Can you work these out from the model? Positions are in its coordinate system, mm. Coordinates: 2 decimals unless noted, no trailing zeros. Write each loop counter-clockwise with the first axis right and the second up, starting at its lowest first coordinate (ties: lowest second). Pieces come first, ordered by that corner, then holes. Notation, with made-up numbers: M 29.5,45.25 L 33.5,45.25 A14 ccw 33.5,64.25 Z; hole C 50.5,65.25 d9. An arc over 180 degrees is marked long. Answer as a JSON object with one key per item and string values. Group by question number.
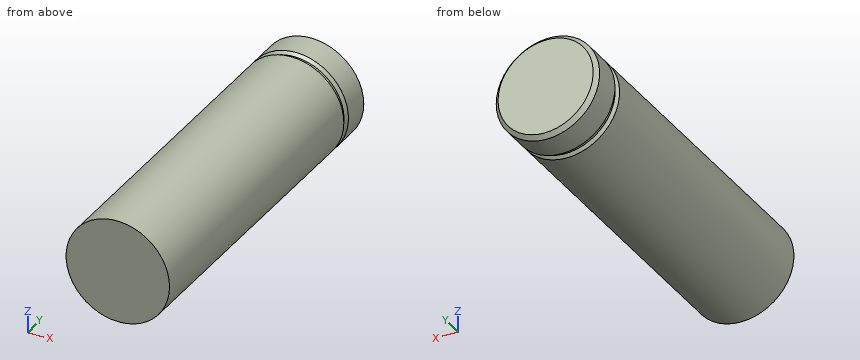
from build123d import *

# Parameters (mm, degrees)
F0_R     = 10
F1_DEPTH = 67.5
F4_SIZE2 = 0.8
F4_SIZE  = 0.8


with BuildPart() as f1:
    # F0 (on Front) → F1 (new body)
    with BuildSketch(Plane.XZ):
        Circle(F0_R)
    extrude(amount=-F1_DEPTH)

    # F2 (on Right) → F3 (revolve, cut)
    with BuildSketch(Plane.YZ):
        Polygon((60.4, 9.455708), (60.9, 9.455708), (61.465685, 10.021394), (59.834315, 10.021394), align=None)
        Polygon((61.465685, -10.021394), (60.9, -9.455708), (60.4, -9.455708), (59.834315, -10.021394), align=None)
    revolve(axis=Axis((0, 0, 0), (0, -1, 0)), mode=Mode.SUBTRACT)

    # F4
    f4_edges = [f1.edges().sort_by_distance(p)[0] for p in [
        (-10, 67.5, 0),
    ]]
    chamfer(f4_edges, length=F4_SIZE, length2=F4_SIZE2)


solid = f1.part
Q1. Will these pins go through, and if not, where does the flat tip stop? pin 1 (6 mm diameter, centred on y = 9, z = -6, fed in from -X); pin 2 (5 mm diameter, centred on x = -7, z = 5.5, fed in from -Y); pin 3 (2 mm diameter, centred on y = 56.5, z = -2.5, fed in from -X); pin 4 (3 mm diameter, centred on y = 15, z = -5.5, fed in from +X).
Q2. If we section it at A-A on y = 26: List the corners of the cut face in (x, z) for me.
Q3. Please list where these lines run through material, in increasing order: L1, parallel to Z at x = -0.5, y = 37; L2, parallel to Z at x = -3.5, y = 14; L3, parallel to X at y = 22, z = -7.5.
Reply:
{
 "1": {"pin 1": "x = -9.54", "pin 2": "y = 0", "pin 3": "x = -9.89", "pin 4": "x = 9.17"},
 "2": {"outline": "C 0,0 d20"},
 "3": {"L1": "-9.99 to 9.99", "L2": "-9.37 to 9.37", "L3": "-6.61 to 6.61"}
}
